Could you check a few things on this drawing? It's one solid part, dimensions in mm from its lowest x, y, z. A direction names the side the tool comes from. Give positions to 0.01 mm unless a question says otherwise; leave off trailing zeros. Loops run counter-clockwise (first coordinate to the right, second up) from the corner with the lowest first, then second, coordinate; pieces in that order, holes last. Notation, with made-up numbers: M 60,-30.75 L 115,-30.75 A18 cw 115,-6.75 Z; hole C 59,50 d4. An arc over 180 degrees is marked long. Return JSON: item names as keys, results as strings. Group by question number.
1. For pin 1 (8 mm diameter, centred on x = 20.5, y = 4, fed in from +Z); pin 2 (11.5 mm diameter, centred on x = 36, z = 91, fed in from -Y); pin 3 (3 mm diameter, centred on x = 162, y = 63.5, fed in from -Z), each with a flat end and sliding along its axis, tell me the tip position at first contact or that it passes through.
2. For the marked faces 4, 5 and 6, which set-ups out of +Z, -Z, +X, -X, +Y, -Y let a thin tool reach every point of the face, with its end or its side?
3. If we section it at D-D (z = 89.5): Write out the boundary of the cut face in (x, y).
4. If we section it at A-A (x = 193): Write out the boundary of the cut face in (y, z), plus the area to 3 significant figures.
5. If we mould it in two halves opening along X, with no side actions, what happens to the marked faces 1, 2 and 3? For each: +X half, -X half, draft (parallel to the pull), parting line (faces both ways), or undercut.
6. If we section it at B-B (y = 67): State how many separate pieces and enclosed holes the cut face has, plus the area to 3 significant figures.
7. Please list where these lines run through material, in increasing order: line 1 (X direction, y = 69, z = 54) (3 decimals); line 2 (Z direction, x = 193, y = 59.5); line 3 (Z direction, x = 183.5, y = 38).
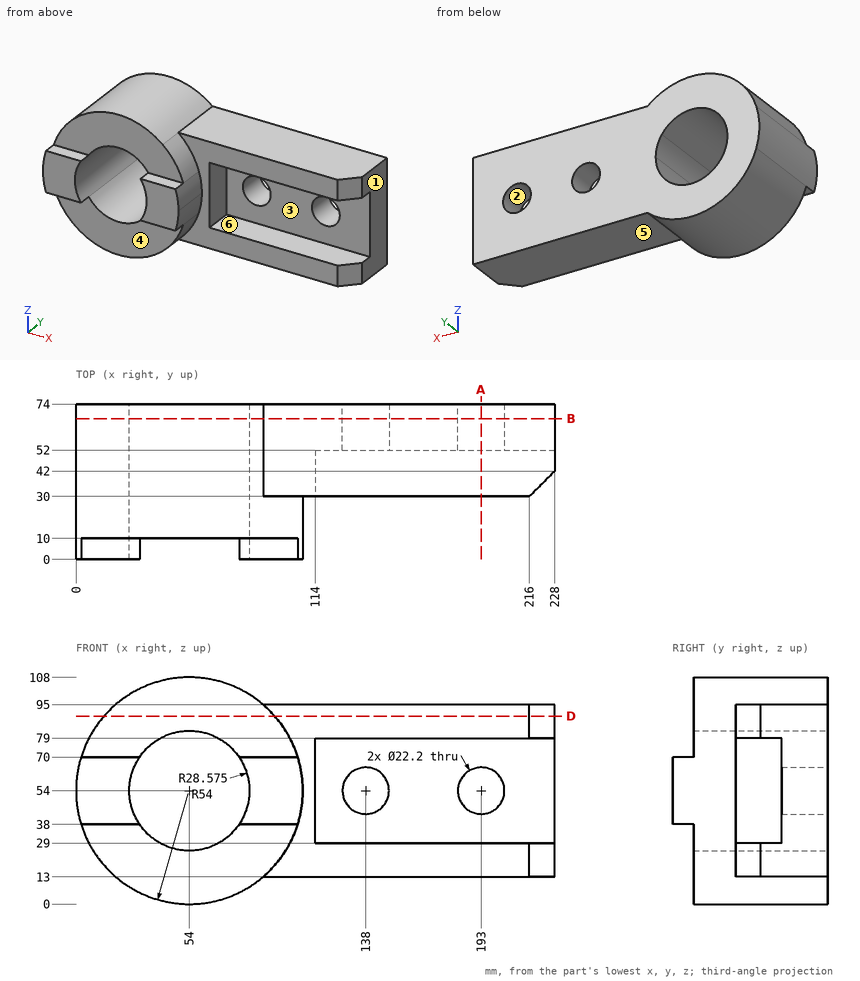
Answer:
{
 "1": {"pin 1": "stops at z = 70", "pin 2": "stops at y = 10", "pin 3": "stops at z = 13"},
 "2": {"face 4": "-Z, +X, -X, -Y", "face 5": "-Z, +X, +Y, -Y", "face 6": "+X, -Y"},
 "3": {"outline": "M 13.31,10 L 94.69,10 L 94.69,30 L 216,30 L 228,42 L 228,74 L 13.31,74 Z"},
 "4": {"outline": "M 30,13 L 74,13 L 74,42.9 L 52,42.9 L 52,29 L 30,29 Z; M 30,79 L 52,79 L 52,65.1 L 74,65.1 L 74,95 L 30,95 Z", "area": "2,020 mm²"},
 "5": {"face 1": "+X half", "face 2": "undercut", "face 3": "draft"},
 "6": {"separate pieces": "1", "enclosed holes": "3", "area": "16,100 mm²"},
 "7": {"line 1": "x = 0 to 25.425, 82.575 to 126.9, 149.1 to 181.9, 204.1 to 228", "line 2": "z = 13 to 42.9, 65.1 to 95", "line 3": "z = 13 to 29, 79 to 95"}
}
